Autodesk Inventor part; units mm, degrees
ref_plane "YZ Plane" through (0, 0, 0) normal (1, 0, 0) x (0, 1, 0)
ref_plane "XZ Plane" through (0, 0, 0) normal (0, 1, 0) x (-1, 0, 0)
ref_plane "XY Plane" through (0, 0, 0) normal (0, 0, 1) x (1, 0, 0)
sketch "Sketch1" plane through (0, 0, 0) normal (0, 0, 1) x (1, 0, 0)
  circle A0 centre (0, 0) radius 12.5
  circle A1 centre (0, 0) radius 25
  line L0 (-25, 0) -> (6, 0)
  line L1 (6, 0) -> (6, -25)
  line L2 (6, -25) -> (-25, -25)
  line L3 (-25, -25) -> (-25, 0)
  line L4 (12.5, 0) -> (12.5, 19.9562)
  line L5 (12.5, 19.9562) -> (8.5, 26.8844)
  line L6 (-4.3412, 24.6202) -> (8.5, 26.8844)
  line L7 (-25, 0) -> (-25, 20.9775)
  line L8 (-25, 20.9775) -> (-4.3412, 24.6202)
  line L9 (-20, -38) -> (0, -38) construction
  point P0 (6, -10.9659)
  point P1 (0, -25)
  point P2 (6, -24.2693)
  point P3 (-12.5, 0)
  dimension "d0" = 25
  dimension "d1" = 50
  dimension "d2" = 6
  dimension "d7" = 150
  dimension "d8" = 4
  dimension "d9" = 110
  dimension "d13" = 38
extrude "Extrusion1" add sketch "Sketch1" along normal mid plane 28 contours A0 L1 L0 | A0 L0 A1 L5 L4 | L0 L1 A0 | A0 L1 A1 L0 | L7 L8 A1 | A1 L2 L3 | L1 L2 A1 | A1 L6 L5
fillet "Fillet1" radius 5 1 edges at (6, -10.9659, 0)
sketch "Sketch2" plane through (0, 0, 0) normal (0, 0, 1) x (1, 0, 0)
  line L0 (8.5, 26.8844) -> (12.5, 19.9562)
  line L1 (12.5, 19.9562) -> (12.5, 0)
  arc A0 (7.8571, -9.7219) -> (12.5, 0) centre (0, 0) ccw
  arc A1 (7.8571, -9.7219) -> (6, -13.6107) centre (11, -13.6107) ccw
  line L2 (6, -13.6107) -> (6, -25)
  line L3 (6, -25) -> (-25, -25)
  line L4 (-25, -25) -> (-25, 20.9775)
  line L5 (-25, 20.9775) -> (8.5, 26.8844)
  line L6 (-25, 20.9775) -> (-44, 17.6273)
  line L7 (-44, 17.6273) -> (-44, -25)
  line L8 (-44, -25) -> (-25, -25)
  line L9 (8.5, 26.8844) -> (-25, 20.9775)
  line L10 (-44, -25) -> (6, -25)
  line L11 (6, -25) -> (6, -38)
  line L12 (6, -38) -> (-44, -38)
  line L13 (-44, -38) -> (-44, -25)
  line L14 (6, -25) -> (6, -13.6107)
  dimension "d14" = 38
  dimension "d21" = 50
extrude "Extrusion2" add sketch "Sketch2" along normal mid plane 18 contours L4 L8 L7 L6 | L3 L11 L12 L13 L8
fillet "Fillet4" radius 8 3 edges at (-25, 20.9775, -11.5) (-25, 20.9775, 11.5) (-44, 17.6273, 0)
fillet "Fillet3" radius 4 2 edges at (-25, -25, 11.5) (-25, -25, -11.5)
chamfer "Chamfer1" distance 2 angle 45 10 edges at (-4.9446, 24.5138, -14) (-23.1284, 19.407, -14) (-25, -3.3677, -14) (-23.8284, -23.8284, -14) (-7.5, -25, -14) (-4.9446, 24.5138, 14) (-23.1284, 19.407, 14) (-25, -3.3677, 14) (-23.8284, -23.8284, 14) (-7.5, -25, 14)
properties part number "Idler Block Left"
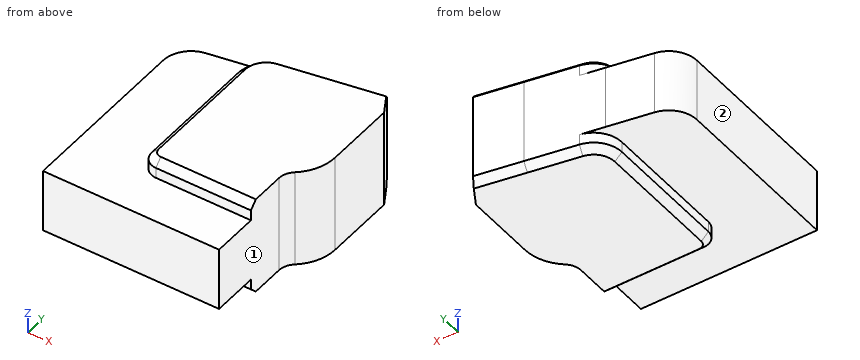
Geometry check sheet. Reference: the model listing, model coordinates, mm. Face numbers are marked on the shaded views. A direction names the side the tool comes from. Coordinates: 2 decimals unless noted, no trailing zeros. Order: outer loops, then holes, each group sorted by start corner. A loop starts at its lowest first (then second) coordinate and runs counter-clockwise, first axis right, second up. Notation, with made-up numbers: (39.5, -20.5) -> (95.5, -20.5) arc R24 cw to (95.5, -4.5) -> close; hole circle Ø9 at (-5, 40.5). An arc over 180 degrees is marked (long way). Use a Markdown table: item, result. Add a question column.
1. Cross-section at A-A (z = 3.75). Enter the section's corners in (x, y).
2. Cross-section at D-D (y = -7.5). Enter the section's corners in (x, z), and give its area (3 significant figures).
3. Go/stop test with flat-tipped pins: pin 1 Ø1.5 at (y, z) = (-7, -11) entering from -X; pin 2 Ø4 at (x, y) = (-27.5, -19.5) entering from -Z; pin 3 Ø1.5 at (x, z) = (-13, 11) entering from -Y. Record where each tip stops, or that it passes through.
4. Cross-section at B-B (y = 7.5). Enter the section's corners in (x, z), and give its area (3 significant figures).
5. Cross-section at C-C (x = -14). Enter the section's corners in (y, z).
6. Set-up check for the marked faces 1 and 2: record each of +Z, -Z, +X, -X, +Y, -Y from which the full face is reachable in a straight line by a thin tool's end or side.
7. Material ranges on L1, parallel to X at y = -18, z = 7.25; L2, parallel to Z at x = -27.5, y = -28.5; L3, parallel to X at y = -16.5, z = 9.5, recorded low to high.
Filled sheet:
| question | item | result |
|---|---|---|
| 1 | outline | (-44, -38) -> (6, -38) -> (6, -13.61) arc R5 cw to (7.86, -9.72) arc R12.5 ccw to (12.5, 0) -> (12.5, 19.96) -> (8.5, 26.88) -> (-4.34, 24.62) -> (-25, 20.98) -> (-37.39, 18.79) arc R8 ccw to (-44, 10.91) -> close |
| 2 | outline | (-44, -9) -> (-25, -9) -> (-25, -12) -> (-23, -14) -> (10, -14) -> (10, 14) -> (-23, 14) -> (-25, 12) -> (-25, 9) -> (-44, 9) -> close |
| 2 | area | 1,320 mm2 |
| 3 | pin 1 | x = -25 |
| 3 | pin 2 | z = -9 |
| 3 | pin 3 | y = -25 |
| 4 | outline | (-44, -9) -> (-25, -9) -> (-25, -12) -> (-23, -14) -> (12.5, -14) -> (12.5, 14) -> (-23, 14) -> (-25, 12) -> (-25, 9) -> (-44, 9) -> close |
| 4 | area | 1,390 mm2 |
| 5 | outline | (-38, -9) -> (-25, -9) -> (-25, -12) -> (-23, -14) -> (20.89, -14) -> (22.92, -12) -> (22.92, 12) -> (20.89, 14) -> (-23, 14) -> (-25, 12) -> (-25, 9) -> (-38, 9) -> close |
| 6 | face 1 | +Z, -Z, +X, -Y |
| 6 | face 2 | +Z, -Z, -X, +Y, -Y |
| 7 | L1 | -44 to 6 |
| 7 | L2 | -9 to 9 |
| 7 | L3 | -25 to 6 |
